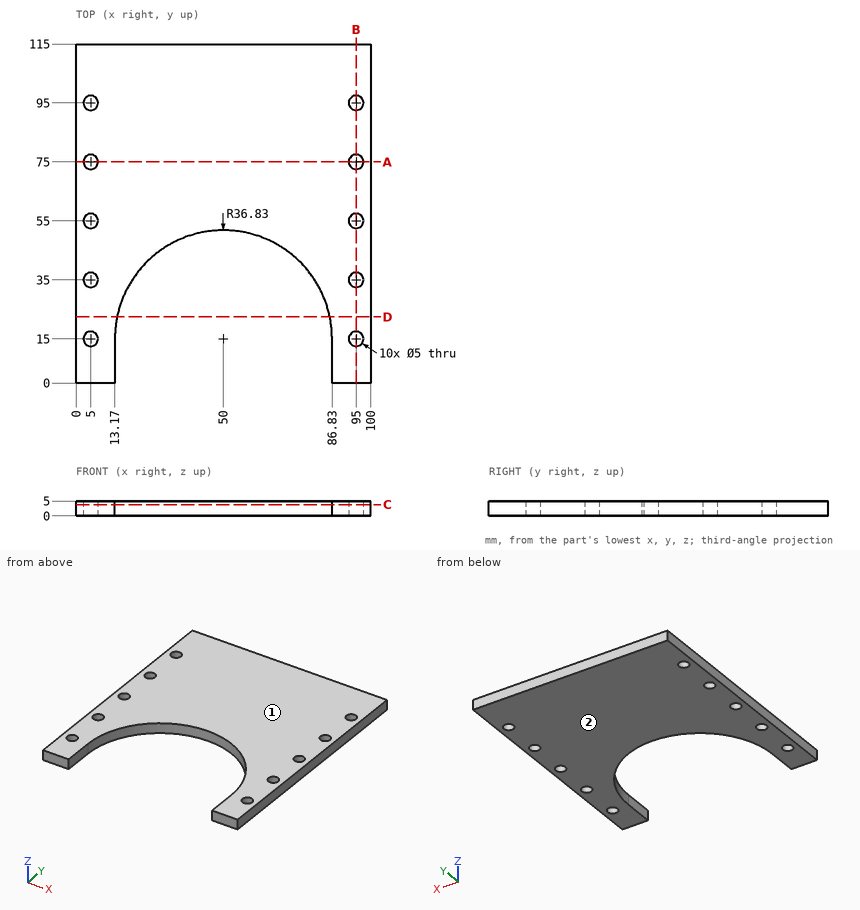
The figure shows three views and two pictorial views of one solid part (mm, origin at its lowest corner). Answer the questions. Round coordinates to 2 decimals unless told otherwise and drop trailing zeros. Write each loop counter-clockwise with the first axis right and the second up, starting at its lowest first coordinate (ties: lowest second). Pieces come first, ordered by that corner, then holes. Notation, with made-up numbers: M 13.5,3 L 39.5,3 A16 ccw 39.5,23 Z; hole C 13,77 d5. An arc over 180 degrees is marked long. Use a Markdown table: item, result.
1) Straight lines are drawn through the part: line 1 along Y through (x, z) = (5, 3.9); line 2 along X through (y, z) = (57, 2.8); line 3 along Y through (x, z) = (73.5, 1.3). For each, find the intervals that lie inside material, in ascending order. Write a range as [from, to].
Answers follow:
| item | result |
|---|---|
| line 1 | y = [0, 12.5], [17.5, 32.5], [37.5, 52.5], [57.5, 72.5], [77.5, 92.5], [97.5, 115] |
| line 2 | x = [0, 3.5], [6.5, 93.5], [96.5, 100] |
| line 3 | y = [43.36, 115] |
2) The part is cut by section C-C (z = 3.8). Give the number of separate pieces and of enclosed holes in the cut face, plus the area to 3 significant figures.
Answers follow:
| item | result |
|---|---|
| separate pieces | 1 |
| enclosed holes | 10 |
| area | 8,070 mm2 |
3) Flat-ended cylindrical pins translate along their axes: pin 1 (4.5 mm diameter, centred on x = 95, y = 15, fed in from -Z); pin 2 (3 mm diameter, centred on x = 25, z = 2.5, fed in from -Y). Find the tip coordinate at first contact, or state that the pin passes through.
Answers follow:
| item | result |
|---|---|
| pin 1 | passes through |
| pin 2 | stops at y = 40.58 |
4) The part is cut by section B-B (x = 95). Write down the section's boundary in (y, z).
Answers follow:
| item | result |
|---|---|
| outline | M 0,0 L 12.5,0 L 12.5,5 L 0,5 Z; M 17.5,0 L 32.5,0 L 32.5,5 L 17.5,5 Z; M 37.5,0 L 52.5,0 L 52.5,5 L 37.5,5 Z; M 57.5,0 L 72.5,0 L 72.5,5 L 57.5,5 Z; M 77.5,0 L 92.5,0 L 92.5,5 L 77.5,5 Z; M 97.5,0 L 115,0 L 115,5 L 97.5,5 Z |
5) For a pull along Z with two mould halves and no side action, classify the marked faces 1 and 2 as pulls with the +Z half, pulls with the -Z half, needs draft (parallel to the pull), parting line crosses it, or undercut.
Answers follow:
| item | result |
|---|---|
| face 1 | pulls with the +Z half |
| face 2 | pulls with the -Z half |
6) The part is cut by section A-A (y = 75). Write down the section's boundary in (x, z).
Answers follow:
| item | result |
|---|---|
| outline | M 0,0 L 2.5,0 L 2.5,5 L 0,5 Z; M 7.5,0 L 92.5,0 L 92.5,5 L 7.5,5 Z; M 97.5,0 L 100,0 L 100,5 L 97.5,5 Z |
7) The part is cut by section D-D (y = 22.5). Write down the section's boundary in (x, z), plus the area to 3 significant figures.
Answers follow:
| item | result |
|---|---|
| outline | M 0,0 L 13.94,0 L 13.94,5 L 0,5 Z; M 86.06,0 L 100,0 L 100,5 L 86.06,5 Z |
| area | 139 mm2 |
